Input: part model. Units: mm. Frame: model coordinates. A direction names the side the tool comes from. Coordinates: 2 decimals unless noted, no trailing zeros. Write each loop counter-clockwise with the first axis right and the second up, starting at its lowest first coordinate (ties: lowest second). Pieces come first, ordered by that corner, then holes. Notation, with made-up numbers: M -32.5,-29 L -19.5,-29 A29 ccw -19.5,-6 Z; hole C 17.5,0 d11. An arc over 180 degrees is marked long. Write each question's results on one line, items separated by ' | '. Start each with the question number.
1. Ray query, probe 1 along X at (y, z) = (-26, 0) (3 decimals); probe 2 along X at (y, z) = (-16, -4.5) (3 decimals); probe 3 along Z at (x, y) = (0, 34). Return the intervals inside material, ascending.
2. First-contact query: pin 1 (3 mm diameter, centred on x = 2, z = -8, fed in from +Y); pin 2 (1 mm diameter, centred on y = 1.5, z = 2.5, fed in from +X); pin 3 (5 mm diameter, centred on y = -21.5, z = -2, fed in from +X) (3 decimals); pin 4 (14 mm diameter, centred on x = -18.75, y = -11.72, fed in from -Z). Flat tips, straight axial feed; report the tip coordinate or a pass-through.
3. Section query C-C, the plane x = 1.5. Output: boundary loops of the cut face in (y, z) (3 decimals), and give its area (3 significant figures).
4. Section query A-A, the plane y = -2. Output: boundary loops of the cut face in (x, z) (3 decimals), and give its area (3 significant figures).
5. Section query D-D, the plane x = -29. Output: boundary loops of the cut face in (y, z), and give its area (3 significant figures).
6. Section query B-B, the plane y = 24. Output: boundary loops of the cut face in (x, z), and give its area (3 significant figures).
7. Set-up query: faces 1 (the flat face through (-9.375, -12, 0)), 2 (the flat face through (-14, -37.5, 0)), 3 (the flat face through (9.375, -18, 0)). Return all of +Z, -Z, +X, -X, +Y, -Y with unobstructed straight access to the full face (end or side cutting, diameter ignored); none if empty.
8. Pull-direction query (Z, two-part tool) for faces 4 (the cylindrical face through (-6.244, 32.319, 0.275)), 5 (the flat face through (-9, 1, -10)), 6 (the flat face through (0, 0, 8)); classes: +Z half, -Z half, draft (parallel to the pull), parting line (faces both ways), or undercut.
```python
from build123d import *

# Parameters (mm, degrees)
F0_W          = 75
F0_H          = 75
F1_DEPTH      = 10
F1_DEPTH_BACK = 10
F3_DEPTH      = 20
F4_R          = 6.25
F5_DEPTH      = 75


# Not quite as in the source:
# - a feature names something its author has since deleted; it is built from what else it names


with BuildPart() as f1:
    # F0 (on Top) → F1 (new body, two sides)
    with BuildSketch(Plane.XY) as f1_sk:
        Rectangle(F0_W, F0_H)
    extrude(amount=F1_DEPTH)
    extrude(f1_sk.sketch, amount=-F1_DEPTH_BACK)

    # F2 (on face) → F3 (cut)
    with BuildSketch(Plane.XY.offset(10)):
        with BuildLine():
            Line((37.5, -37.5), (37.5, 18.75))
            add(Edge.make_bspline(
                [(9.375, 0), (18.75, 6.25), (18.75, 18.75), (37.5, 18.75)],
                knots=[0, 0, 0, 0, 33.8020432075, 33.8020432075, 33.8020432075, 33.8020432075], degree=3))
            Line((9.375, 0), (9.375, -37.5))
            Line((9.375, -37.5), (18.75, -37.5))
            Line((18.75, -37.5), (37.5, -37.5))
        make_face()
        with BuildLine():
            ThreePointArc((0, 37.5), (20.9631372891, 32.5512745781), (37.5, 18.75))
            Line((37.5, 18.75), (37.5, 37.5))
            Line((37.5, 37.5), (0, 37.5))
        make_face()
        with BuildLine():
            ThreePointArc((-37.5, 18.75), (-20.9631372891, 32.5512745781), (0, 37.5))
            Line((0, 37.5), (-37.5, 37.5))
            Line((-37.5, 37.5), (-37.5, 18.75))
        make_face()
        with BuildLine():
            Line((0, -28.125), (4.6875, -32.8125))
            add(Edge.make_bspline(
                [(4.6875, -32.8125), (3.6620711894, -24.6951237234), (2.6366423788, -16.5777474468), (3.0432450075, -9.375)],
                knots=[0, 0, 0, 0, 0.3697687561, 0.3697687561, 0.3697687561, 0.3697687561], degree=3))
            Line((3.0432450075, -9.375), (-3.0432450075, -9.375))
            add(Edge.make_bspline(
                [(-4.6875, -32.8125), (-3.6620711894, -24.6951237234), (-2.6366423788, -16.5777474468), (-3.0432450075, -9.375)],
                knots=[0, 0, 0, 0, 0.3697687561, 0.3697687561, 0.3697687561, 0.3697687561], degree=3))
            Line((-4.6875, -32.8125), (0, -28.125))
        make_face()
        with BuildLine():
            Line((-9.375, -18.75), (-9.375, -4.6875))
            ThreePointArc((-9.375, -4.6875), (-25.78125, -2.34375), (-28.125, -18.75))
            ThreePointArc((-28.125, -18.75), (-18.75, -23.4375), (-9.375, -18.75))
        make_face()
        with BuildLine():
            Line((-4.6875, 0), (4.6875, 0))
            add(Edge.make_bspline(
                [(4.6875, 0), (7.2279380084, 7.6213140251), (12.9889690042, 13.1856570125), (18.75, 18.75)],
                knots=[0.5419601085, 0.5419601085, 0.5419601085, 0.5419601085, 1, 1, 1, 1], degree=3))
            ThreePointArc((18.75, 18.75), (0, 28.1290022772), (-18.75, 18.75))
            add(Edge.make_bspline(
                [(-4.6875, 0), (-7.2279380084, 7.6213140251), (-12.9889690042, 13.1856570125), (-18.75, 18.75)],
                knots=[0.5419601085, 0.5419601085, 0.5419601085, 0.5419601085, 1, 1, 1, 1], degree=3))
        make_face()
    extrude(amount=-F3_DEPTH, mode=Mode.SUBTRACT)

    # F4 (on face) → F5 (cut)
    with BuildSketch(Plane.XZ.offset(37.5)):
        Circle(F4_R)
    extrude(amount=-F5_DEPTH, mode=Mode.SUBTRACT)


solid = f1.part
```
Answer:
1) probe 1: -37.5 to -6.25, 6.25 to 9.375 | probe 2: -37.5 to -29.659, -9.375 to -4.337, 4.337 to 9.375 | probe 3: -10 to -6.25, 6.25 to 10
2) pin 1: y = 37.5 | pin 2: x = 11.89 | pin 3: x = 9.375 | pin 4: through
3) outline: M -37.5,-10 L -29.625,-10 L -29.625,-6.067 L -37.5,-6.067 Z; M -37.5,6.067 L -29.625,6.067 L -29.625,10 L -37.5,10 Z; M -9.375,-10 L 0,-10 L 0,-6.067 L -9.375,-6.067 Z; M -9.375,6.067 L 0,6.067 L 0,10 L -9.375,10 Z; M 28.081,-10 L 37.476,-10 L 37.476,-6.067 L 28.081,-6.067 Z; M 28.081,6.067 L 37.476,6.067 L 37.476,10 L 28.081,10 Z | area: 210 mm^2
4) outline: M -37.5,-10 L -25.298,-10 L -25.298,10 L -37.5,10 Z; M -12.202,-10 L 9.375,-10 L 9.375,10 L -12.202,10 Z; hole C 0,0 d12.5 | area: 553 mm^2
5) outline: M -37.5,-10 L -17.4,-10 L -17.4,10 L -37.5,10 Z; M -6.04,-10 L 27.45,-10 L 27.45,10 L -6.04,10 Z | area: 1,070 mm^2
6) outline: M -32.91,-10 L -13.28,-10 L -13.28,10 L -32.91,10 Z; M 13.28,-10 L 32.91,-10 L 32.91,10 L 13.28,10 Z | area: 785 mm^2
7) face 1: +Z, -Z | face 2: +Z, -Z, +X, -X, -Y | face 3: +Z, -Z, +X, -Y
8) face 4: undercut | face 5: -Z half | face 6: draft
